Read the model definition and answer for the solid it produces. Units are mm, in the model's axes. Face numbers are marked on the shaded views. A direction names the side the tool comes from. Give positions to 0.01 mm unless a question says otherwise; leave off trailing zeros. Loops run counter-clockwise (first coordinate to the right, second up) from the corner with the lowest first, then second, coordinate; pieces in that order, holes last. Notation, with made-up numbers: (74, -17) - (123, -17) arc R28 ccw to (123, 9) - close; hole circle Ø9 at (0, 71). An arc over 180 degrees is marked (long way). Put each result on its own line as item: value. Start each with the question number.
1. A cutting plane is placed at B-B, the plane z = 0. Determine the outline of the cut face in (x, y), plus the area to 3 significant figures.
2. For the marked faces 1, 2 and 3, determine the directions among +Z, -Z, +X, -X, +Y, -Y from which every point of the face is accessible in a straight line to the end or side of a thin tool.
3. A cutting plane is placed at C-C, the plane y = 51. Determine the outline of the cut face in (x, z).
4. Consider L1, parallel to Y at x = 2.5, z = -4; L2, parallel to X at y = 23.5, z = 0.25; L3, parallel to X at y = 33, z = 1. Determine where each line is inside the solid, lowest interval first. Write a range as from..to.
5. A cutting plane is placed at A-A, the plane x = 0. Determine the outline of the cut face in (y, z).
6. Given pin 1 Ø3 at (x, y) = (-3.5, 47) entering from +Z; pin 2 Ø5 at (x, z) = (0, 0.5) entering from -Y; pin 3 Ø2 at (x, y) = (3.5, 55.5) entering from +Z; pin 4 Ø1.5 at (x, z) = (-3, 2.5) entering from -Y, each flat-ended and moving along its own axis, determine where each tip first touches the part or whether it passes through.
7. A cutting plane is placed at D-D, the plane y = 19. Determine the outline of the cut face in (x, z), plus the area to 3 significant figures.
Autodesk Inventor part; units mm, degrees
ref_plane "YZ Plane" through (0, 0, 0) normal (1, 0, 0) x (0, 1, 0)
ref_plane "XZ Plane" through (0, 0, 0) normal (0, 1, 0) x (-1, 0, 0)
ref_plane "XY Plane" through (0, 0, 0) normal (0, 0, 1) x (1, 0, 0)
sketch "Эскиз1" plane through (0, 0, 0) normal (0, 1, 0) x (-1, 0, 0)
  circle A0 centre (0, 0) radius 2.5
  dimension "d0" = 5
extrude "Выдавливание1" add sketch "Эскиз1" along normal blind 85
thread "Резьба1"
ref_plane "РабПлоскость1" through (0, 42.5, 0) normal (0, -1, 0) x (1, 0, 0)
sketch "Эскиз2" plane through (0, 42.5, 0) normal (0, -1, 0) x (1, 0, 0)
  circle A0 centre (0, 0) radius 5
  dimension "d5" = 10
extrude "Выдавливание2" add sketch "Эскиз2" along normal blind 10 and the other way blind 20
properties part number "Screw"
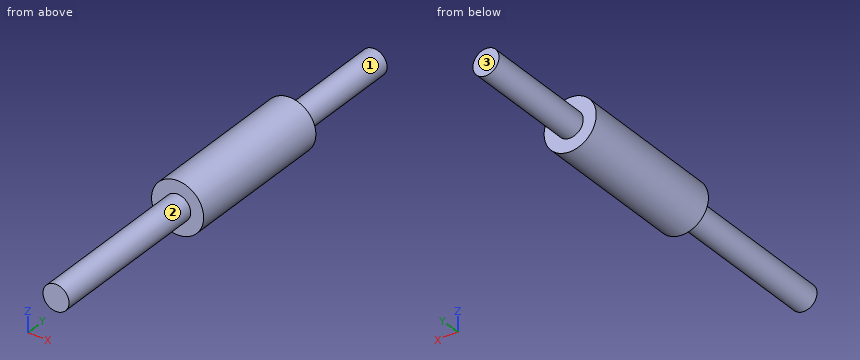
Return value:
1. outline: (-5, 32.5) - (-2.5, 32.5) - (-2.5, 0) - (2.5, 0) - (2.5, 32.5) - (5, 32.5) - (5, 62.5) - (2.5, 62.5) - (2.5, 85) - (-2.5, 85) - (-2.5, 62.5) - (-5, 62.5) - close
1. area: 575 mm2
2. face 1: +Y
2. face 2: -Y
2. face 3: +Z, -Z, +X, -X, +Y
3. outline: circle Ø10 at (0, 0)
4. L1: y = 32.5..62.5
4. L2: x = -2.49..2.49
4. L3: x = -4.9..4.9
5. outline: (0, -2.5) - (32.5, -2.5) - (32.5, -5) - (62.5, -5) - (62.5, -2.5) - (85, -2.5) - (85, 2.5) - (62.5, 2.5) - (62.5, 5) - (32.5, 5) - (32.5, 2.5) - (0, 2.5) - close
6. pin 1: stops at z = 4.58
6. pin 2: stops at y = 0
6. pin 3: stops at z = 4.33
6. pin 4: stops at y = 32.5
7. outline: circle Ø5 at (0, 0)
7. area: 19.6 mm2
